The listing builds one solid part. Answer for the finished solid, in the listing's coordinates (mm). Face numbers are marked on the shaded views. Give positions to 0.01 mm unless a question says otherwise; leave off trailing zeros. Write each loop counter-clockwise with the first axis right and the second up, starting at its lowest first coordinate (ties: lowest second). Pieces come first, ordered by that corner, then holes. Notation, with made-up numbers: (35, 31) - (59, 31) arc R24 cw to (59, 52) - close; hole circle Ø2 at (80, 54). An arc over 180 degrees is marked (long way). One line per question, with ' | ' between items. Start each with the question number.
1. Find the intervals of material crossed by L1, parallel to Y at x = 0, z = -5.5; L2, parallel to X at y = 1.5, z = -1.5; L3, parallel to X at y = 1, z = -1.5, in increasing order. Write a range as from..to.
2. The mould has two halves that part along X. Classify the marked faces 1, 2, 3 and 4: +X half, -X half, draft (parallel to the pull), parting line (faces both ways), or undercut.
3. A cutting plane is placed at C-C (z = -8). Determine the outline of the cut face in (x, y), then the cut area to 3 significant figures.
4. A cutting plane is placed at A-A (x = 0). Determine the outline of the cut face in (y, z), then the cut area to 3 significant figures.
```python
from build123d import *

# Parameters (mm, degrees)
IZIM1_W            = 90
IZIM1_H            = 90
IZIM1_R            = 7.25
TABAN_FLAN_1_DEPTH = 10
RADYUS1_R          = 10


# Sheet-metal steps are written as plain solids
with BuildPart() as part:
    # Çizim1 → Taban-Flanş1 (new body)
    with BuildSketch(Plane.XY):
        Rectangle(IZIM1_W, IZIM1_H)
        Circle(IZIM1_R, mode=Mode.SUBTRACT)
    extrude(amount=-TABAN_FLAN_1_DEPTH)

    # Radyus1
    radyus1_edges = [part.edges().sort_by_distance(p)[0] for p in [
        (45, -45, -5),
        (-45, -45, -5),
        (-45, 45, -5),
        (45, 45, -5),
    ]]
    fillet(radyus1_edges, radius=RADYUS1_R)


solid = part.part
```
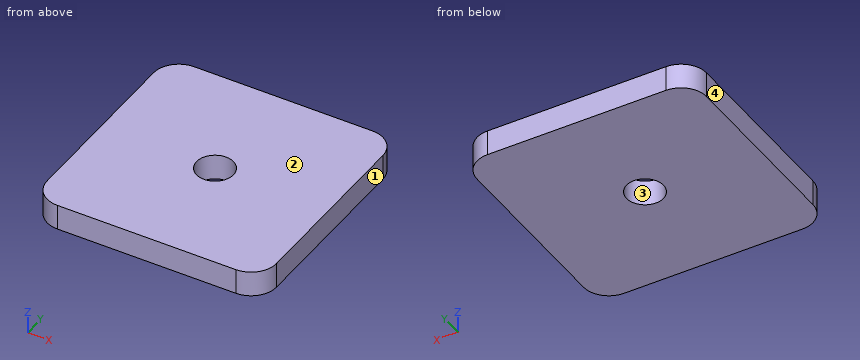
Determined:
1) L1: -45..-7.25, 7.25..45 | L2: -45..-7.09, 7.09..45 | L3: -45..-7.18, 7.18..45
2) face 1: +X half | face 2: draft | face 3: undercut | face 4: -X half
3) outline: (-45, -35) arc R10 ccw to (-35, -45) - (35, -45) arc R10 ccw to (45, -35) - (45, 35) arc R10 ccw to (35, 45) - (-35, 45) arc R10 ccw to (-45, 35) - close; hole circle Ø14.5 at (0, 0) | area: 7,850 mm2
4) outline: (-45, -10) - (-7.25, -10) - (-7.25, 0) - (-45, 0) - close; (7.25, -10) - (45, -10) - (45, 0) - (7.25, 0) - close | area: 755 mm2
